Could you check a few things on this model? Use its own coordinates, in mm. Face numbers are marked on the shaded views. A direction names the side the tool comes from. Coordinates: 2 decimals unless noted, no trailing zeros. Order: outer loops, then holes, each group sorted by start corner. A loop starts at its lowest first (then second) coordinate and runs counter-clockwise, first axis right, second up. Notation, with made-up numbers: (51.5, -31.5) - (103.5, -31.5) arc R21 cw to (103.5, 1.5) - close; hole circle Ø1 at (6, 50.25). An arc over 180 degrees is marked (long way). One line per item, written item: value.
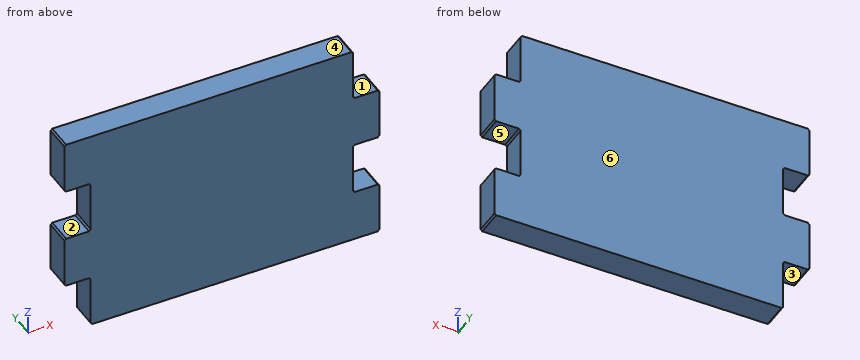
from build123d import *

# Parameters (mm, degrees)
F1_DEPTH = 12.7
F2_SIZE  = 0.79375


# Not quite as in the source:
# - a feature names something its author has since deleted; it is built from what else it names


with BuildPart() as f1:
    # F0 (on Front) → F1 (new body)
    with BuildSketch(Plane.XZ):
        Polygon((-63.5, 25.4508), (-63.5, 0), (76.2, 0), (76.2, 25.4), (63.5, 25.4), (63.5, 51.0032), (76.2, 51.0032), (76.2, 76.4032), (63.5, 76.4032), (63.5, 101.854), (-76.2, 101.854), (-76.2, 76.454), (-63.5, 76.454), (-63.5, 50.8508), (-76.2, 50.8508), (-76.2, 25.4508), align=None)
    extrude(amount=F1_DEPTH)

    # F2
    f2_edges = [f1.edges().sort_by_distance(p)[0] for p in [
        (-63.5, -6.35, 76.454),
        (-63.5, -6.35, 50.8508),
        (-63.5, -6.35, 25.4508),
        (-63.5, -6.35, 0),
        (63.5, -6.35, 101.854),
        (76.2, -6.35, 76.4032),
        (63.5, -6.35, 76.4032),
        (63.5, -6.35, 25.4),
        (76.2, -6.35, 25.4),
        (76.2, -6.35, 51.0032),
        (63.5, -6.35, 51.0032),
        (-76.2, -6.35, 50.8508),
        (-76.2, -6.35, 25.4508),
        (76.2, -6.35, 0),
        (-76.2, -6.35, 101.854),
        (-76.2, -6.35, 76.454),
    ]]
    chamfer(f2_edges, length=F2_SIZE)


solid = f1.part
Item 1: If I drill on probe 1 along X at (y, z) = (-1.5, 84); probe 2 along X at (y, z) = (-9, 5); probe 3 along Z at (x, y) = (63, -5.5), over which ranges is the centre line in solid material (lowest first)?
Conclusion:
probe 1: -76.2 to 63.5
probe 2: -63.5 to 76.2
probe 3: 0 to 101.56
Item 2: Thinking about a two-plate mould opening in Z: for the marked faces 4, 5 and 6, which applies, pulls with the +Z half, pulls with the -Z half, needs draft (parallel to the pull), parting line crosses it, or undercut?
Conclusion:
face 4: pulls with the +Z half
face 5: undercut
face 6: needs draft
Item 3: I'm going to push flat-ended pins straight in: pin 1 Ø3.5 at (x, y) = (-69.5, -8) entering from -Z; pin 2 Ø6.5 at (y, z) = (-4, 65) entering from -X; pin 3 Ø5.5 at (x, y) = (72, -9.5) entering from +Z. Where does each tip first touch, or does it pass through?
Conclusion:
pin 1: z = 25.45
pin 2: x = -63.5
pin 3: z = 76.4
Item 4: I want a section at B-B on z = 8. Please give me the cut outline in (x, y), then the cut area to 3 significant figures.
Conclusion:
outline: (-63.5, -12.7) - (76.2, -12.7) - (76.2, 0) - (-63.5, 0) - close
area: 1,770 mm²
Item 5: For the marked faces 1, 2 and 3, which set-ups out of +Z, -Z, +X, -X, +Y, -Y let a thin tool reach every point of the face, with its end or its side?
Conclusion:
face 1: +Z, +X, +Y, -Y
face 2: -X, +Y, -Y
face 3: -Z, -X, +Y, -Y
